from build123d import *

# Parameters (mm, degrees)
SKETCH1_R           = 20
SKETCH1_R_2         = 15
BOSS_EXTRUDE1_DEPTH = 10
SKETCH3_W           = 40
SKETCH3_H           = 40
BOSS_EXTRUDE2_DEPTH = 5
SKETCH5_R           = 15
CUT_EXTRUDE1_DEPTH  = 5
SKETCH7_W           = 14.853626256
SKETCH7_H           = 40
BOSS_EXTRUDE3_DEPTH = 35
FILLET1_R           = 5
FILLET2_R           = 5
SKETCH8_R           = 3
CUT_EXTRUDE2_DEPTH  = 35
SKETCH9_W           = 10.266740892
SKETCH9_H           = 48.673472914
CUT_EXTRUDE5_DEPTH  = 35


with BuildPart() as part:
    # Sketch1 → Boss-Extrude1 (new body)
    with BuildSketch(Plane(origin=(0, 0, 0), x_dir=(1, 0, 0), z_dir=(0, 1, 0))):
        with Locations(Location((0, 0, 0), (0, 0, 270))):
            Circle(SKETCH1_R)
        with Locations(Location((0, 0, 0), (0, 0, 270))):
            Circle(SKETCH1_R_2, mode=Mode.SUBTRACT)
    extrude(amount=BOSS_EXTRUDE1_DEPTH)

    # Sketch3 → Boss-Extrude2 (add)
    with BuildSketch(Plane(origin=(0, 10, 0), x_dir=(1, 0, 0), z_dir=(0, 1, 0))):
        Rectangle(SKETCH3_W, SKETCH3_H)
    extrude(amount=BOSS_EXTRUDE2_DEPTH)

    # Sketch5 → Cut-Extrude1 (cut)
    with BuildSketch(Plane.XZ.offset(-10)):
        with Locations(Location((0, 0, 0), (0, 0, 270))):
            Circle(SKETCH5_R)
    extrude(amount=-CUT_EXTRUDE1_DEPTH, mode=Mode.SUBTRACT)

    # Sketch7 → Boss-Extrude3 (add)
    with BuildSketch(Plane(origin=(0, 15, 0), x_dir=(1, 0, 0), z_dir=(0, 1, 0))):
        Rectangle(SKETCH7_W, SKETCH7_H)
    extrude(amount=BOSS_EXTRUDE3_DEPTH)

    # Fillet1
    fillet1_edges = [part.edges().sort_by_distance(p)[0] for p in [
        (0, 50, 20),
    ]]
    fillet(fillet1_edges, radius=FILLET1_R)

    # Fillet2
    fillet2_edges = [part.edges().sort_by_distance(p)[0] for p in [
        (0, 50, -20),
    ]]
    fillet(fillet2_edges, radius=FILLET2_R)

    # Sketch8 → Cut-Extrude2 (cut)
    with BuildSketch(Plane(origin=(7.426813128, 0, 0), x_dir=(0, 0, -1), z_dir=(1, 0, 0))):
        with Locations((-14.80323114, 44.772968188)):
            Circle(SKETCH8_R)
        with Locations((14.80323114, 44.772968188)):
            Circle(SKETCH8_R)
    extrude(amount=-CUT_EXTRUDE2_DEPTH, mode=Mode.SUBTRACT)

    # Sketch9 → Cut-Extrude5 (cut)
    with BuildSketch(Plane(origin=(0, 50, 0), x_dir=(1, 0, 0), z_dir=(0, 1, 0))):
        Rectangle(SKETCH9_W, SKETCH9_H)
    extrude(amount=-CUT_EXTRUDE5_DEPTH, mode=Mode.SUBTRACT)


solid = part.part
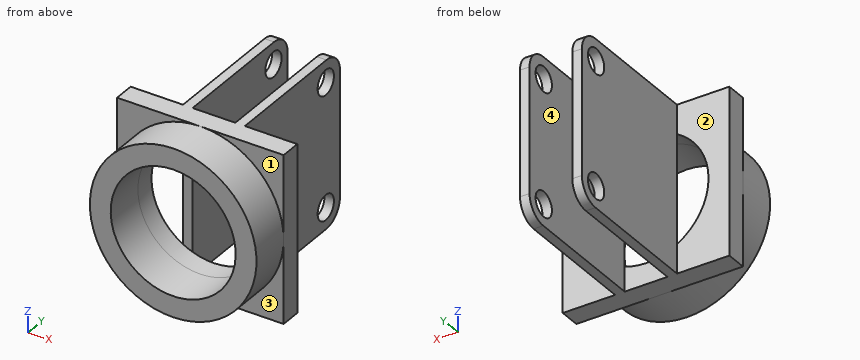
The model under review builds one solid part; all positions refer to its coordinate system, in mm. Face numbers are marked on the shaded views. A direction names the side the tool comes from. Round coordinates to 2 decimals unless told otherwise and drop trailing zeros. Loops run counter-clockwise (first coordinate to the right, second up) from the corner with the lowest first, then second, coordinate; pieces in that order, holes last. Notation, with made-up numbers: M 29.5,34 L 54.5,34 A31 cw 54.5,70 Z; hole C -33,-39 d1. An arc over 180 degrees is marked long. Answer as CSV lines item,"result". Start each with the question number.
Item 1: For the marked faces 1, 2, 3 and 4, list the 3-axis set-ups (+Z, -Z, +X, -X, +Y, -Y) from which the entire face can be reached by the end or side of a thin tool; tool diameter is ignored.
Item 2: Insertion check: P1, Ø6, axis at x = -8, z = 13, coming from the -Y side; P2, Ø1, axis at y = 38.5, z = -10, coming from the -X side; P3, Ø4.5, axis at x = 2.5, z = -17.5, coming from the +Y side; P4, Ø10.5, axis at y = 34, z = -3.5, coming from the +X side. Each pin has a flat end and moves straight along its axis. Give the tip position at first contact, or say it passes through.
Item 3: Consider section C-C (z = -3). Write out the cut boundary in (x, y), then the cut area to 3 significant figures.
Item 4: Consider section B-B (x = 12). Write out the cut boundary in (y, z).
Item 5: Consider section D-D (x = 2). Write out the cut boundary in (y, z), then the cut area to 3 significant figures.
Item 6: Consider section A-A (y = 25.5). Write out the cut boundary in (x, z).
Item 7: Wall thickness on line 1 (X direction, y = 37, z = 16.5); line 2 (Z direction, x = 0, y = 3); line 3 (Y direction, x = -12, z = -11.5): over which ranges is each line inside the solid? List them lowest first. Write a range as [from, to].
Answer:
1,face 1,"+Z, +X, -Y"
1,face 2,"+Z, -Z, -X, +Y"
1,face 3,"-Z, +X, -Y"
1,face 4,"+Z, -Z, +Y"
2,P1,"stops at y = 0"
2,P2,"stops at x = -7.43"
2,P3,"stops at y = 15"
2,P4,"stops at x = 7.43"
3,outline,"M -20,10 L -19.77,10 L -19.77,0 L -14.7,0 L -14.7,15 L -20,15 Z; M -7.43,15 L -5.13,15 L -5.13,50 L -7.43,50 Z; M 5.13,15 L 7.43,15 L 7.43,50 L 5.13,50 Z; M 14.7,0 L 19.77,0 L 19.77,10 L 20,10 L 20,15 L 14.7,15 Z"
3,area,"315 mm^2"
4,outline,"M 0,-16 L 10,-16 L 10,-20 L 15,-20 L 15,-9 L 0,-9 Z; M 0,9 L 15,9 L 15,20 L 10,20 L 10,16 L 0,16 Z"
5,outline,"M 0,-19.9 L 10,-19.9 L 10,-20 L 15,-20 L 15,-14.87 L 0,-14.87 Z; M 0,14.87 L 15,14.87 L 15,20 L 10,20 L 10,19.9 L 0,19.9 Z"
5,area,"152 mm^2"
6,outline,"M -7.43,-20 L -5.13,-20 L -5.13,20 L -7.43,20 Z; M 5.13,-20 L 7.43,-20 L 7.43,20 L 5.13,20 Z"
7,line 1,"x = [-7.43, -5.13], [5.13, 7.43]"
7,line 2,"z = [-20, -15], [15, 20]"
7,line 3,"y = [0, 15]"
